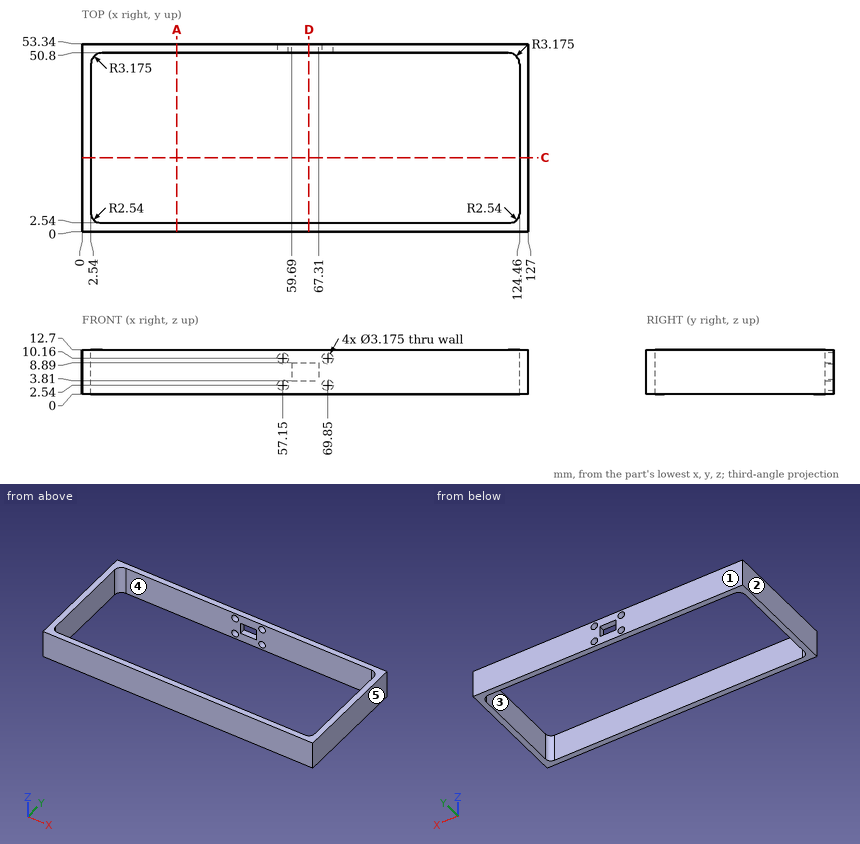
Source: three-view drawing plus pictorial views. Frame: mm from the lowest corner of the part. A direction names the side the tool comes from. Round coordinates to 2 decimals unless told otherwise and drop trailing zeros. Order: outer loops, then holes, each group sorted by start corner. A loop starts at its lowest first (then second) coordinate and runs counter-clockwise, first axis right, second up. Notation, with made-up numbers: (22.25, 43) - (58.25, 43) arc R29 cw to (58.25, 71) - close; hole circle Ø3 at (6.25, -30). An arc over 180 degrees is marked (long way). Answer in a Markdown table with one row per item.
Item 1: Section query C-C (y = 21). Return the cut outline in (x, z), then the cut area to 3 significant figures.
Model answer:
| item | result |
|---|---|
| outline | (0, 0) - (2.54, 0) - (2.54, 12.7) - (0, 12.7) - close; (124.46, 0) - (127, 0) - (127, 12.7) - (124.46, 12.7) - close |
| area | 64.5 mm² |
Item 2: Reachability of the marked faces 4 and 5 from +Z, -Z, +X, -X, +Y, -Y: full face, straight path, thin tool, end or side. Return the list, or none.
Model answer:
| item | result |
|---|---|
| face 4 | +Z, -Z |
| face 5 | +Z, -Z, +X, +Y, -Y |
Item 3: Section query D-D (x = 64.5). Return the cut outline in (y, z), then the cut area to 3 significant figures.
Model answer:
| item | result |
|---|---|
| outline | (0, 0) - (2.54, 0) - (2.54, 12.7) - (0, 12.7) - close; (50.8, 0) - (53.34, 0) - (53.34, 3.81) - (50.8, 3.81) - close; (50.8, 8.89) - (53.34, 8.89) - (53.34, 12.7) - (50.8, 12.7) - close |
| area | 51.6 mm² |
Item 4: Line query: line 1 (Z direction, x = 57, y = 52); line 2 (X direction, y = 52.25, z = 2.54); line 3 (X direction, y = 9.5, z = 3.25). Output: solid intervals per line, ascending.
Model answer:
| item | result |
|---|---|
| line 1 | z = 0 to 0.96, 4.12 to 8.58, 11.74 to 12.7 |
| line 2 | x = 0 to 55.56, 58.74 to 68.26, 71.44 to 127 |
| line 3 | x = 0 to 2.54, 124.46 to 127 |
Item 5: Section query A-A (x = 27). Return the cut outline in (y, z).
Model answer:
| item | result |
|---|---|
| outline | (0, 0) - (2.54, 0) - (2.54, 12.7) - (0, 12.7) - close; (50.8, 0) - (53.34, 0) - (53.34, 12.7) - (50.8, 12.7) - close |
Item 6: Mould query, pull axis X, two halves, no side actions, for the marked faces 1, 2 and 3. Classes: released by +X, released by -X, zero draft, split by the parting line, or undercut.
Model answer:
| item | result |
|---|---|
| face 1 | zero draft |
| face 2 | released by -X |
| face 3 | undercut |
